Answer from the drawing. Dimensions are ordinates in mm from the lowest x, y and z of the part. A direction names the side the tool comes from. Coordinates: 2 decimals unless noted, no trailing zeros. Order: outer loops, then holes, each group sorted by start corner. A loop starts at its lowest first (then second) coordinate and runs counter-clockwise, first axis right, second up. Notation, with made-up numbers: (15, 57) -> (32, 57) arc R16 cw to (32, 64) -> close; hole circle Ø5 at (18.25, 28.5). An arc over 180 degrees is marked (long way). Use CSV: the item, a comma, the result in double quotes.
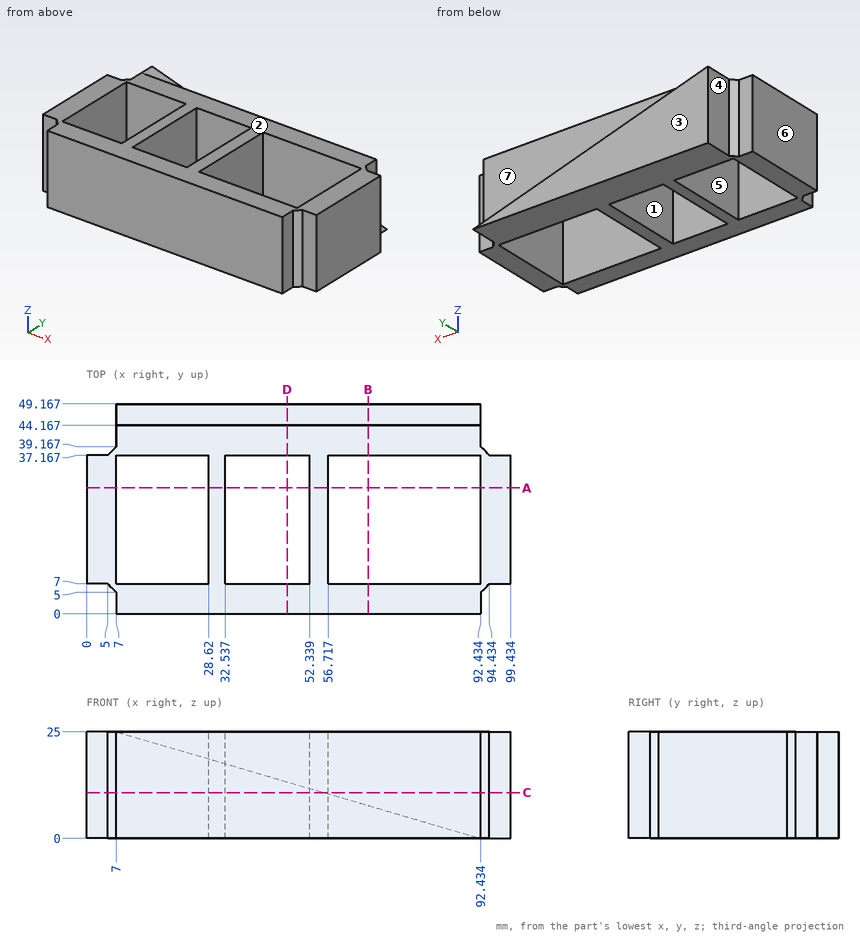
Item 1: Find section D-D, the plane x = 47. Give the vertices of the cut face in (y, z) (1 decimal).
Return value:
outline,"(0, 0) -> (7, 0) -> (7, 25) -> (0, 25) -> close; (37.2, 0) -> (49.2, 0) -> (49.2, 13.3) -> (44.2, 13.3) -> (44.2, 25) -> (37.2, 25) -> close"
Item 2: Find section A-A, the plane y = 29.5. Give the vertices of the cut face in (x, z).
Return value:
outline,"(0, 0) -> (7, 0) -> (7, 25) -> (0, 25) -> close; (28.62, 0) -> (32.54, 0) -> (32.54, 25) -> (28.62, 25) -> close; (52.34, 0) -> (56.72, 0) -> (56.72, 25) -> (52.34, 25) -> close; (92.43, 0) -> (99.43, 0) -> (99.43, 25) -> (92.43, 25) -> close"
Item 3: Straight lines are drawn through the part: line 1 along X through (y, z) = (32.5, 5); line 2 along Y through (x, z) = (69, 14.5); line 3 along Y through (x, z) = (25.5, 11.5). For each, find the intervals that lie inside material, in ascending order.
Return value:
line 1,"x = 0 to 7, 28.62 to 32.54, 52.34 to 56.72, 92.43 to 99.43"
line 2,"y = 0 to 7, 37.17 to 44.17"
line 3,"y = 0 to 7, 37.17 to 49.17"
Item 4: Each of these flat-tipped pins is pushed along its axis until it touches: P1, Ø2, axis at x = 68, y = 9, coming from the -Z side; P2, Ø4, axis at y = 2, z = 7, coming from the +X side; P3, Ø5.5, axis at x = 1.5, z = 17, coming from the -Y side; P4, Ø11, axis at y = 43.5, z = 10.5, coming from the -X side (1 decimal). Where does it stop, or does it pass through?
Return value:
P1,"passes through"
P2,"stops at x = 92.43"
P3,"stops at y = 7"
P4,"stops at x = 5.8"
Item 5: Find section C-C, the plane z = 10.75. Give the number of separate pieces and of enclosed holes in the cut face, then the cut area to 3 significant figures.
Return value:
separate pieces,"1"
enclosed holes,"3"
area,"2,120 mm^2"
Item 6: The mould has two halves that part along Y. Classify the marked faces 1, 2 and 3: +Y half, -Y half, draft (parallel to the pull), parting line (faces both ways), or undercut.
Return value:
face 1,"undercut"
face 2,"draft"
face 3,"+Y half"
Item 7: A tool of negligible diameter and unlimited length cuts with its end or side. For the marked faces 4, 5, 6 and 7, from which of +Z, -Z, +X, -X, +Y, -Y can it reach the whole face along a straight path? Write none if from no direction.
Return value:
face 4,"+Z, -Z, -X, +Y"
face 5,"+Z, -Z"
face 6,"+Z, -Z, -X, +Y, -Y"
face 7,"+Z, +X, +Y"
Item 8: Find section B-B, the plane x = 66. Give the vertices of the cut face in (y, z) (1 decimal), then the cut area to 3 significant figures.
Return value:
outline,"(0, 0) -> (7, 0) -> (7, 25) -> (0, 25) -> close; (37.2, 0) -> (49.2, 0) -> (49.2, 7.7) -> (44.2, 7.7) -> (44.2, 25) -> (37.2, 25) -> close"
area,"389 mm^2"
